Check sheet for the modelled part. Datum: model origin and axes. Units: mm. A direction names the side the tool comes from. Give positions to 0.01 mm unless a question says otherwise; leave off trailing zeros. Loops run counter-clockwise (first coordinate to the right, second up) from the corner with the lowest first, then second, coordinate; pieces in that order, holes last. Notation, with made-up numbers: (23, -14) - (60, -14) arc R15 cw to (60, 11) - close; hole circle Ø1 at (23.25, 2.5). An arc over 180 degrees is marked (long way). Use CSV: the item, a comma, the result in double quotes.
from build123d import *

# Parameters (mm, degrees)
SKETCH1_W                   = 27.69
SKETCH1_H                   = 63.625
F_7_8_0_88_DIAMETER_HOLE1_D = 22.352
CIRPATTERN1_COUNT           = 8


with BuildPart() as part:
    # Sketch1 → Revolve1 (revolve)
    with BuildSketch(Plane.XY):
        Polygon((239.01, 68.795), (266.7, 68.795), (266.7, 74.295), (239.01, 74.295), (81.28, 74.295), (0, 50.18683312), (0, 44.45), (82.078476138, 68.795), align=None)
        with Locations((252.855, 106.1075)):
            Rectangle(SKETCH1_W, SKETCH1_H)
    revolve(axis=Axis((0, 0, 0), (1, 0, 0)))

    # 7/8 (0.88) Diameter Hole1 (through all)
    with Locations(Plane(origin=(266.7, 111.466065597, 46.170756115), x_dir=(0, 0, 1), z_dir=(1, 0, 0))):
        with Locations((0, 0)):
            f_7_8_0_88_diameter_hole1 = Hole(F_7_8_0_88_DIAMETER_HOLE1_D / 2)

    # CirPattern1: 7/8 (0.88) Diameter Hole1 ×8 about axis
    cirpattern1_axis = Axis((0, 0, 0), (1, 0, 0))
    for i in range(1, CIRPATTERN1_COUNT):
        add(f_7_8_0_88_diameter_hole1.rotate(cirpattern1_axis, i * 360 / CIRPATTERN1_COUNT), mode=Mode.SUBTRACT)


solid = part.part
1. Go/stop test with flat-tipped pins: pin 1 Ø3 at (x, y) = (138, -50) entering from +Z; pin 2 Ø18 at (y, z) = (46.17, -111.47) entering from +X; pin 3 Ø6 at (x, z) = (101, 45) entering from -Y; pin 4 Ø1.5 at (x, z) = (122.5, -51) entering from -Y. Record where each tip stops, or that it passes through.
Completed:
pin 1,"stops at z = 56.28"
pin 2,"passes through"
pin 3,"stops at y = -61.28"
pin 4,"stops at y = -54.72"
2. Sectioned sample at C-C, the plane x = 196. Record the boundary of the cut face in (y, z) (3 decimals).
Completed:
outline,"circle Ø148.59 at (0, 0); hole circle Ø137.59 at (0, 0)"
3. Set-up check for faces 1 (the face through (0, -30, -33.2)), 2 (the face through (239.01, -59, -59)): record each of +Z, -Z, +X, -X, +Y, -Y from which the full face is reachable in a straight line by a thin tool's end or side.
Completed:
face 1,"+Z, -Z, -X, +Y, -Y"
face 2,"-X"
4. Sectioned sample at D-D, the plane z = -118. Record the boundary of the cut face in (x, y).
Completed:
outline,"(239.01, -71.4) - (266.7, -71.4) - (266.7, -55.24) - (239.01, -55.24) - close; (239.01, -37.1) - (266.7, -37.1) - (266.7, 37.1) - (239.01, 37.1) - close; (239.01, 55.24) - (266.7, 55.24) - (266.7, 71.4) - (239.01, 71.4) - close"
5. Scan lines: line 1 along X through (y, z) = (-100, -2.5); line 2 along Z through (x, y) = (201.5, -6.5); line 3 along Y through (x, z) = (126, -51). Record each from-to range of solid material in increasing order.
Completed:
line 1,"x = 239.01 to 266.7"
line 2,"z = -74.01 to -68.49, 68.49 to 74.01"
line 3,"y = -54.03 to -46.17, 46.17 to 54.03"
6. Sectioned sample at A-A, the plane z = 0. Record the boundary of the cut face in (x, y) (3 decimals).
Completed:
outline,"(0, -50.187) - (81.28, -74.295) - (239.01, -74.295) - (239.01, -137.92) - (266.7, -137.92) - (266.7, -68.795) - (82.078, -68.795) - (0, -44.45) - close; (0, 44.45) - (82.078, 68.795) - (266.7, 68.795) - (266.7, 137.92) - (239.01, 137.92) - (239.01, 74.295) - (81.28, 74.295) - (0, 50.187) - close"
7. Release check for a two-part mould opening along Y. For faces 3 (the face through (175.68, 65.62, 20.66)), 4 (the face through (159.041, -58.958, -45.207)), 5 (the face through (266.7, -29, 63)) record: released by +Y, released by -Y, zero draft, split by the parting line, or undercut.
Completed:
face 3,"undercut"
face 4,"split by the parting line"
face 5,"zero draft"
